Work out the finished part from the listing and answer in its coordinate system (mm). A direction names the side the tool comes from. Coordinates: 2 decimals unless noted, no trailing zeros. Order: outer loops, then holes, each group sorted by start corner. A loop starts at its lowest first (then second) coordinate and runs counter-clockwise, first axis right, second up. Notation, with made-up numbers: M 69,-35 L 128,-35 A20 cw 128,-30 Z; hole C 36.5,-39.75 d6. An arc over 180 degrees is marked long. Answer in a Markdown table with one row per item. Add a question column.
Item 1: Consider line 1 (Y direction, x = -17, z = 3.75); line 2 (Z direction, x = -26, y = 2.55); line 3 (Z direction, x = -26.5, y = 0.75). Determine where each line is inside the solid, lowest interval first. Write a range as from..to.
Item 2: The part is cut by section D-D (x = -1.5). Write down the section's boundary in (y, z), then the cut area to 3 significant figures.
Item 3: The part is cut by section B-B (z = 11.25). Write down the section's boundary in (x, y), then the cut area to 3 significant figures.
Item 4: Flat-ended cylindrical pins translate along their axes: pin 1 Ø2.5 at (x, z) = (-12.5, 8.5) entering from +Y; pin 2 Ø2 at (y, z) = (-6, 2) entering from -X; pin 3 Ø8 at (x, z) = (4.5, 9) entering from -Y; pin 4 Ø4 at (x, z) = (-26, 5) entering from -Y. Find the tip coordinate at first contact, or state that the pin passes through.
Item 5: The part is cut by section A-A (z = -1). Write down the section's boundary in (x, y), then the cut area to 3 significant figures.
Item 6: The part is cut by section C-C (x = 6). Write down the section's boundary in (y, z).
Item 7: Which of the six approach directions +Z, -Z, +X, -X, +Y, -Y give full straight-line access (tool end or side, diameter ignored) to faces 1 (the face through (-27, -5.5, -1)), 2 (the face through (9, 4, 2.5)), 3 (the face through (-27, 3.5, -1))?
from build123d import *

# Parameters (mm, degrees)
F0_W      = 10
F0_H      = 2
F0_W_2    = 2
F1_DEPTH  = 2
F2_DEPTH  = 12
F4_DEPTH  = 25
F5_DEPTH  = 3
F7_R      = 1.5
F8_DEPTH  = 1
F9_SIZE   = 4
F10_SIZE  = 4
F11_DEPTH = 2.5
F13_DEPTH = 20
F14_SIZE  = 1
F15_W     = 3
F15_H     = 2
F16_DEPTH = 1


with BuildPart() as f1:
    # F0 (on Top) → F1 (new body)
    with BuildSketch(Plane.XY):
        with Locations((-14, -6.5)):
            Rectangle(F0_W, F0_H)
        with Locations((-14, 6.5)):
            Rectangle(F0_W, F0_H)
        Polygon((-30, 7.5), (-30, -7.5), (-19, -7.5), (-19, -5.5), (-19, -3.5), (-9, -3.5), (-9, -5.5), (-9, -7.5), (30, -7.5), (30, 7.5), (-9, 7.5), (-9, 5.5), (-9, 3.5), (-19, 3.5), (-19, 5.5), (-19, 7.5), align=None)
        with Locations((-27, -4.5)):
            Rectangle(F0_W_2, F0_H, mode=Mode.SUBTRACT)
        with Locations((27, -4.5)):
            Rectangle(F0_W_2, F0_H, mode=Mode.SUBTRACT)
        with Locations((-27, 4.5)):
            Rectangle(F0_W_2, F0_H, mode=Mode.SUBTRACT)
        Polygon((3, 3.5), (3, -3.5), (23, -3.5), (23, -7), (3, -7), (3, -6.5), (0, -6.5), (0, 6.5), (3, 6.5), (3, 7), (23, 7), (23, 3.5), align=None, mode=Mode.SUBTRACT)
        with Locations((27, 4.5)):
            Rectangle(F0_W_2, F0_H, mode=Mode.SUBTRACT)
        with Locations((-14, 4.5)):
            Rectangle(F0_W, F0_H)
        with Locations((-14, -4.5)):
            Rectangle(F0_W, F0_H)
        Polygon((3, 6.5), (3, 3.5), (23, 3.5), (23, 7), (3, 7), align=None)
        Polygon((23, -3.5), (3, -3.5), (3, -6.5), (3, -7), (23, -7), align=None)
        Polygon((3, -6.5), (3, -3.5), (3, 3.5), (3, 6.5), (0, 6.5), (0, -6.5), align=None)
    extrude(amount=-F1_DEPTH)

    # F0 (on Top) → F2 (join)
    with BuildSketch(Plane.XY):
        with Locations((-14, 4.5)):
            Rectangle(F0_W, F0_H)
        with Locations((-14, -4.5)):
            Rectangle(F0_W, F0_H)
    extrude(amount=F2_DEPTH)

    # F3 (on face) → F4 (cut)
    with BuildSketch(Plane(origin=(0, 5.5, 0), x_dir=(-1, 0, 0), z_dir=(0, 1, 0))):
        with BuildLine():
            Line((14, 7), (14, 10))
            ThreePointArc((14, 10), (12.5, 8.5), (14, 7))
        make_face()
        with BuildLine():
            ThreePointArc((14, 7), (15.0606601718, 7.4393398282), (15.5, 8.5))
            ThreePointArc((15.5, 8.5), (15.0606601718, 9.5606601718), (14, 10))
            Line((14, 10), (14, 7))
        make_face()
    extrude(amount=-F4_DEPTH, mode=Mode.SUBTRACT)

    # F0 (on Top) → F5 (join)
    with BuildSketch(Plane.XY):
        with Locations((-14, 6.5)):
            Rectangle(F0_W, F0_H)
        with Locations((-14, -6.5)):
            Rectangle(F0_W, F0_H)
    extrude(amount=F5_DEPTH)

    # F7 (on offset) → F8 (join, symmetric)
    with BuildSketch(Plane.XZ.offset(-3)):
        with BuildLine():
            ThreePointArc((-30, 5), (-26, 1), (-22, 5))
            ThreePointArc((-22, 5), (-26, 9), (-30, 5))
        make_face()
        with Locations((-26, 5)):
            Circle(F7_R, mode=Mode.SUBTRACT)
        with BuildLine():
            Line((-22, 0), (-22, 5))
            ThreePointArc((-22, 5), (-26, 1), (-30, 5))
            Line((-30, 5), (-30, 0))
            Line((-30, 0), (-22, 0))
        make_face()
    extrude(amount=F8_DEPTH, both=True)

    # F9
    f9_edges = [f1.edges().sort_by_distance(p)[0] for p in [
        (-9, 4.5, 12),
        (-19, 4.5, 12),
    ]]
    chamfer(f9_edges, length=F9_SIZE)

    # F10
    f10_edges = [f1.edges().sort_by_distance(p)[0] for p in [
        (-9, -4.5, 12),
        (-19, -4.5, 12),
    ]]
    chamfer(f10_edges, length=F10_SIZE)

    # F0 (on Top) → F11 (join)
    with BuildSketch(Plane.XY):
        Polygon((23, -3.5), (3, -3.5), (3, -6.5), (3, -7), (23, -7), align=None)
        Polygon((3, 6.5), (3, 3.5), (23, 3.5), (23, 7), (3, 7), align=None)
        Polygon((3, -6.5), (3, -3.5), (3, 3.5), (3, 6.5), (0, 6.5), (0, -6.5), align=None)
    extrude(amount=F11_DEPTH)

    # F12 (on face) → F13 (cut)
    with BuildSketch(Plane.YZ.offset(23)):
        Polygon((-3.5, 2.5), (-5.25, 0), (-3.5, 0), align=None)
        Polygon((-7, 0.5), (-5.25, 2.5), (-7, 2.5), align=None)
        Polygon((7, 0.5), (7, 2.5), (5.25, 2.5), align=None)
        Polygon((5.25, 0), (3.5, 2.5), (3.5, 0), align=None)
    extrude(amount=-F13_DEPTH, mode=Mode.SUBTRACT)

    # F14
    f14_edges = [f1.edges().sort_by_distance(p)[0] for p in [
        (1.5, 6.5, 2.5),
        (1.5, -6.5, 2.5),
    ]]
    chamfer(f14_edges, length=F14_SIZE)

    # F15 (on face) → F16 (cut)
    with BuildSketch(Plane.XY.offset(2.5)):
        with Locations((1.5, 0)):
            Rectangle(F15_W, F15_H)
    extrude(amount=-F16_DEPTH, mode=Mode.SUBTRACT)


solid = f1.part
Reply:
| question | item | result |
|---|---|---|
| 1 | line 1 | y = -5.5..-3.5, 3.5..5.5 |
| 1 | line 2 | z = -2..3.5, 6.5..9 |
| 1 | line 3 | z = -2..0 |
| 2 | outline | M -7.5,-2 L 7.5,-2 L 7.5,0 L -7.5,0 Z |
| 2 | area | 30.0 mm2 |
| 3 | outline | M -15.75,-5.5 L -12.25,-5.5 L -12.25,-3.5 L -15.75,-3.5 Z; M -15.75,3.5 L -12.25,3.5 L -12.25,5.5 L -15.75,5.5 Z |
| 3 | area | 14.0 mm2 |
| 4 | pin 1 | stops at y = 5.5 |
| 4 | pin 2 | stops at x = -19 |
| 4 | pin 3 | passes through |
| 4 | pin 4 | stops at y = 2 |
| 5 | outline | M -30,-7.5 L 30,-7.5 L 30,7.5 L -30,7.5 Z; hole M -28,-5.5 L -26,-5.5 L -26,-3.5 L -28,-3.5 Z; hole M -28,3.5 L -26,3.5 L -26,5.5 L -28,5.5 Z; hole M 26,-5.5 L 28,-5.5 L 28,-3.5 L 26,-3.5 Z; hole M 26,3.5 L 28,3.5 L 28,5.5 L 26,5.5 Z |
| 5 | area | 884 mm2 |
| 6 | outline | M -7.5,-2 L 7.5,-2 L 7.5,0 L 7,0 L 7,0.5 L 5.25,2.5 L 3.5,2.5 L 5.25,0 L -5.25,0 L -3.5,2.5 L -5.25,2.5 L -7,0.5 L -7,0 L -7.5,0 Z |
| 7 | face 1 | +Z, -Z |
| 7 | face 2 | +Z, +X, +Y, -Y |
| 7 | face 3 | -Z |
